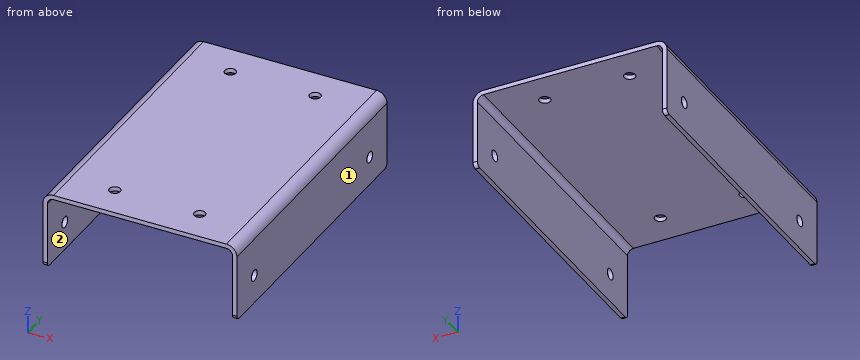
Autodesk Inventor part; units mm, degrees
ref_plane "YZ Plane" through (0, 0, 0) normal (1, 0, 0) x (0, 1, 0)
ref_plane "XZ Plane" through (0, 0, 0) normal (0, 1, 0) x (-1, 0, 0)
ref_plane "XY Plane" through (0, 0, 0) normal (0, 0, 1) x (1, 0, 0)
sketch "Sketch1" plane through (0, 0, 0) normal (0, 0, 1) x (1, 0, 0)
  line L0 (-42, 0) -> (42, 0)
  line L1 (42, 0) -> (42, -130)
  line L2 (42, -130) -> (-42, -130)
  line L3 (-42, -130) -> (-42, 0)
  point P0 (0, 0)
  point P1 (0, 0)
  dimension "d0" = 84
  dimension "d1" = 130
extrude "Plate1" add sketch "Sketch1" along normal blind 2
sketch "Sketch2" plane through (42, -130, 0) normal (1, 0, 0) x (0, 1, 0)
  line L0 (130, 0) -> (0, 0)
  line L1 (0, 0) -> (0, -33)
  line L2 (0, -33) -> (130, -33)
  line L3 (130, -33) -> (130, 0)
edge flange "Flange1" height 35 angle 90 thickness 2 bend radius 2.75 thickness toward (1, 0, 0) relief round relief width 2 relief depth 1 corner gap 2.75 corner form 0 edges at (42, -65, 0) (-42, -65, 0) wall of the first edge with corners at (42, 0, 0) (42, -130, 0) (42, -130, -33) (42, 0, -33)
bend "Bend1"
corner "Corner1"
sketch "Sketch3" plane through (0, 0, 0) normal (1, 0, 0) x (0, 1, 0)
  line L0 (0, -33) -> (-130, -33)
  line L1 (-115, -20) -> (-115, -20) construction
  line L2 (-117.5, -20) -> (-117.5, -20)
  line L3 (-112.5, -20) -> (-112.5, -20)
  arc A0 (-112.5, -20) -> (-117.5, -20) centre (-115, -20) ccw
  arc A1 (-117.5, -20) -> (-112.5, -20) centre (-115, -20) ccw
  line L4 (-130, -2.75) -> (-130, -33)
  point P0 (0, 0)
  point P1 (-115, -20)
  dimension "d14" = 0
  dimension "d15" = 13
  dimension "d17" = 2.5
  dimension "d18" = 15
extrude "Extrusion1" cut sketch "Sketch3" along normal through all both and the other way through all
sketch "Sketch6" plane through (0, 0, 2) normal (0, 0, 1) x (1, 0, 0)
  line L0 (-39.25, 0) -> (39.25, 0)
  circle A0 centre (19.25, -115) radius 2.5
  line L1 (44, -112.5) -> (44, -117.5)
  circle A1 centre (-19.25, -115) radius 2.5
  line L2 (39.25, -130) -> (39.25, 0)
  line L3 (0, 0) -> (0, -130) construction
  line L4 (-39.25, -130) -> (39.25, -130)
  point P0 (0, 0)
  point P1 (44, -115)
  dimension "d27" = 5
  dimension "d33" = 20
extrude "Extrusion3" cut sketch "Sketch6" against normal blind 10
fillet "Fillet1" radius 2 4 edges at (43, 0, -33) (-43, 0, -33) (43, -130, -33) (-43, -130, -33)
pattern_linear "Rectangular Pattern2" count 2 spacing 100 along (0, 1, 0) of "Extrusion1", "Extrusion3"
equation "\"d2\" = Thickness"
equation "\"d3\" = BendReliefWidth"
equation "\"d4\" = BendReliefDepth"
equation "\"d5\" = MinimumRemnant"
equation "\"d6\" = TransitionRadius"
equation "\"d9\" = BendRadius"
equation "\"d10\" = CornerReliefSize"
equation "\"d11\" = GapSize"
equation "\"d12\" = JacobiRadiusSize"
equation "\"BendReliefWidth\" = Thickness"
equation "\"BendReliefDepth\" = 0.5 * Thickness"
equation "\"CornerReliefSize\" = 4 * Thickness"
equation "\"MinimumRemnant\" = 2 * Thickness"
equation "\"TransitionRadius\" = BendRadius"
equation "\"JacobiRadiusSize\" = BendRadius"
equation "\"GapSize\" = Thickness"
properties part number "NDM 11.029 bracket 29" material "Stainless Steel"
Read the model definition and answer for the solid it produces. Units are mm, in the model's axes. Face numbers are marked on the shaded views. A direction names the side the tool comes from. Give positions to 0.01 mm unless a question says otherwise; leave off trailing zeros. Write each loop counter-clockwise with the first axis right and the second up, starting at its lowest first coordinate (ties: lowest second). Pieces come first, ordered by that corner, then holes. Notation, with made-up numbers: (3, 24) - (9, 24) arc R18 ccw to (9, 45) - close; hole circle Ø6 at (33.25, 24.25). An arc over 180 degrees is marked (long way). Return JSON: item names as keys, results as strings.
Q1. For the marked faces 1 and 2, determine the directions among +Z, -Z, +X, -X, +Y, -Y from which every point of the face is accessible in a straight line to the end or side of a thin tool.
Reply:
{"face 1": "+Z, -Z, +X, +Y, -Y", "face 2": "-Z, +Y, -Y"}
Q2. Consider line 1 along Y through (x, z) = (19.25, 1.4); line 2 along X through (y, z) = (-65.5, -14.5); line 3 along Z through (x, y) = (22, -33). Determine where each line is inside the solid, lowest interval first. Write a range as [from, to].
Reply:
{"line 1": "[-130, -117.5], [-112.5, -17.5], [-12.5, 0]", "line 2": "[-44, -42], [42, 44]", "line 3": "[0, 2]"}
Q3. A cutting plane is placed at D-D, the plane z = -6.5. Determine the outline of the cut face in (x, y), and give its area (3 significant figures).
Reply:
{"outline": "(-44, -130) - (-42, -130) - (-42, 0) - (-44, 0) - close; (42, -130) - (44, -130) - (44, 0) - (42, 0) - close", "area": "520 mm²"}
Q4. A cutting plane is placed at A-A, the plane y = -115. Determine the outline of the cut face in (x, z), and give its area (3 significant figures).
Reply:
{"outline": "(-44, -33) - (-42, -33) - (-42, -22.5) - (-44, -22.5) - close; (-44, -17.5) - (-42, -17.5) - (-42, -2.75) arc R2.75 cw to (-39.25, 0) - (-21.75, 0) - (-21.75, 2) - (-39.25, 2) arc R4.75 ccw to (-44, -2.75) - close; (-16.75, 0) - (16.75, 0) - (16.75, 2) - (-16.75, 2) - close; (21.75, 0) - (39.25, 0) arc R2.75 cw to (42, -2.75) - (42, -17.5) - (44, -17.5) - (44, -2.75) arc R4.75 ccw to (39.25, 2) - (21.75, 2) - close; (42, -33) - (44, -33) - (44, -22.5) - (42, -22.5) - close", "area": "262 mm²"}
Q5. Given P1, Ø6.5, axis at x = 19.25, y = -15, coming from the -Z side; P2, Ø12, axis at x = 34.5, y = -33.5, coming from the -Z side, each flat-ended and moving along its own axis, determine where each tip first touches the part or whether it passes through.
Reply:
{"P1": "z = 0", "P2": "z = -0.3"}
Q6. A cutting plane is placed at C-C, the plane x = -19.25. Determine the outline of the cut face in (y, z), and give its area (3 significant figures).
Reply:
{"outline": "(-130, 0) - (-117.5, 0) - (-117.5, 2) - (-130, 2) - close; (-112.5, 0) - (-17.5, 0) - (-17.5, 2) - (-112.5, 2) - close; (-12.5, 0) - (0, 0) - (0, 2) - (-12.5, 2) - close", "area": "240 mm²"}
Q7. A cutting plane is placed at B-B, the plane z = -20. Determine the outline of the cut face in (x, y).
Reply:
{"outline": "(-44, -130) - (-42, -130) - (-42, -117.5) - (-44, -117.5) - close; (-44, -112.5) - (-42, -112.5) - (-42, -17.5) - (-44, -17.5) - close; (-44, -12.5) - (-42, -12.5) - (-42, 0) - (-44, 0) - close; (42, -130) - (44, -130) - (44, -117.5) - (42, -117.5) - close; (42, -112.5) - (44, -112.5) - (44, -17.5) - (42, -17.5) - close; (42, -12.5) - (44, -12.5) - (44, 0) - (42, 0) - close"}
